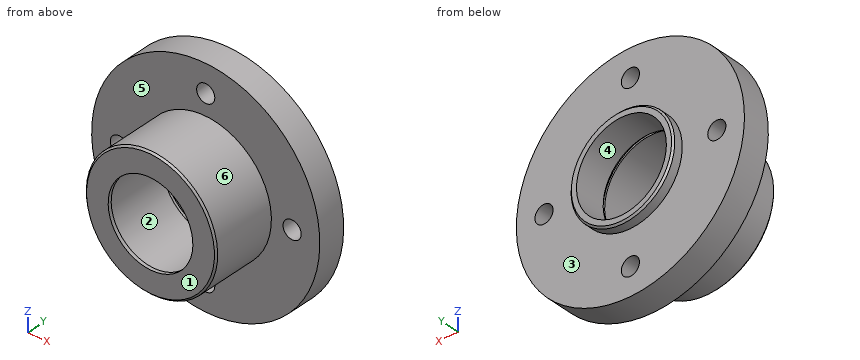
from build123d import *

# Parameters (mm, degrees)
OTW_R_GWINTOWANY_M12X1_51_D = 10.5


with BuildPart() as part:
    # Szkic1 → Obrót1 (revolve)
    with BuildSketch(Plane.XY, mode=Mode.PRIVATE) as obr_t1_sk:
        Polygon((30, 80.923148938), (66, 80.923148938), (66, 64.923148938), (38, 64.923148938), (38, 39.923148938), (38, 28.923148938), (37, 27.923148938), (24.5, 27.923148938), (24.5, 29.923148938), (27, 29.923148938), (27, 66.923148938), (28, 66.923148938), (28, 69.073148938), (26, 69.073148938), (26, 80.923148938), (26, 86.923148938), (29, 86.923148938), (30, 85.923148938), align=None)
    revolve(obr_t1_sk.sketch.rotate(Axis((0, 0, 0), (0, 1, 0)), 90), axis=Axis((0, 0, 0), (0, 1, 0)))

    # Otwór gwintowany M12x1.51 (through all)
    with Locations(Plane(origin=(-50, 80.923148938, 0), x_dir=(0, 0, 1), z_dir=(0, 1, 0))):
        with Locations((0, 0), (-50, 50), (0, 100), (50, 50)):
            Hole(OTW_R_GWINTOWANY_M12X1_51_D / 2)


solid = part.part
Geometry check sheet. Reference: the model listing, model coordinates, mm. Face numbers are marked on the shaded views. A direction names the side the tool comes from. Coordinates: 2 decimals unless noted, no trailing zeros. Order: outer loops, then holes, each group sorted by start corner. A loop starts at its lowest first (then second) coordinate and runs counter-clockwise, first axis right, second up. Notation, with made-up numbers: (-31.5, 82) -> (26.5, 82) arc R24 cw to (26.5, 92) -> close; hole circle Ø5 at (15, -25.75). An arc over 180 degrees is marked (long way). Use a Markdown table: item, result. Add a question column.
1. Cross-section at B-B (x = 47.5). Enter the section's corners in (y, z).
2. Set-up check for the marked faces 1, 2 and 3: record each of +Z, -Z, +X, -X, +Y, -Y from which the full face is reachable in a straight line by a thin tool's end or side.
3. Cross-section at A-A (y = 76.5). Enter the section's corners in (x, z).
4. Go/stop test with flat-tipped pins: pin 1 Ø1 at (y, z) = (62.5, 3.5) entering from -X; pin 2 Ø13.5 at (x, z) = (0, 50) entering from -Y; pin 3 Ø17 at (x, z) = (-50, 0) entering from +Y. Record where each tip stops, or that it passes through.
5. Cross-section at C-C (z = 50). Enter the section's corners in (x, y), and give its area (3 significant figures).
6. Mould release check, pull along X, two halves, no side actions. Record for the marked faces 4, 5 and 6: pulls with the +X half, pulls with the -X half, needs draft (parallel to the pull), parting line crosses it, or undercut.
7. Material ranges on L1, parallel to X at y = 71, z = 0; L2, parallel to X at y = 58, z = 0; L3, parallel to X at y = 78, z = -3.5, recorded low to high.
8. Cross-section at D-D (x = 0). Give the number of separate pieces and of enclosed holes in the cut face, and give its area (3 significant figures).
Filled sheet:
| question | item | result |
|---|---|---|
| 1 | outline | (64.92, -45.82) -> (80.92, -45.82) -> (80.92, -4.62) -> (64.92, -4.62) -> close; (64.92, 4.62) -> (80.92, 4.62) -> (80.92, 45.82) -> (64.92, 45.82) -> close |
| 2 | face 1 | +Z, -Z, +X, -X, -Y |
| 2 | face 2 | none |
| 2 | face 3 | +Y |
| 3 | outline | circle Ø132 at (0, 0); hole circle Ø10.5 at (-50, 0); hole circle Ø52 at (0, 0); hole circle Ø10.5 at (0, -50); hole circle Ø10.5 at (0, 50); hole circle Ø10.5 at (50, 0) |
| 4 | pin 1 | x = -37.88 |
| 4 | pin 2 | y = 64.92 |
| 4 | pin 3 | y = 80.92 |
| 5 | outline | (-43.08, 64.92) -> (-5.25, 64.92) -> (-5.25, 80.92) -> (-43.08, 80.92) -> close; (5.25, 64.92) -> (43.08, 64.92) -> (43.08, 80.92) -> (5.25, 80.92) -> close |
| 5 | area | 1,210 mm2 |
| 6 | face 4 | undercut |
| 6 | face 5 | needs draft |
| 6 | face 6 | parting line crosses it |
| 7 | L1 | -66 to -55.25, -44.75 to -26, 26 to 44.75, 55.25 to 66 |
| 7 | L2 | -38 to -27, 27 to 38 |
| 7 | L3 | -65.91 to -53.91, -46.09 to -25.76, 25.76 to 46.09, 53.91 to 65.91 |
| 8 | separate pieces | 4 |
| 8 | enclosed holes | 0 |
| 8 | area | 1,800 mm2 |
